The listing builds one solid part. Answer for the finished solid, in the listing's coordinates (mm). Face numbers are marked on the shaded views. Round coordinates to 2 decimals unless told otherwise and drop trailing zeros. Order: outer loops, then holes, each group sorted by start corner. A loop starts at its lowest first (then second) coordinate and runs counter-clockwise, first axis right, second up. Notation, with made-up numbers: (86, 72.25) - (104, 72.25) arc R26 ccw to (104, 101.25) - close; hole circle Ø4 at (51.25, 25). An arc over 180 degrees is marked (long way). Write item = value, one per line.
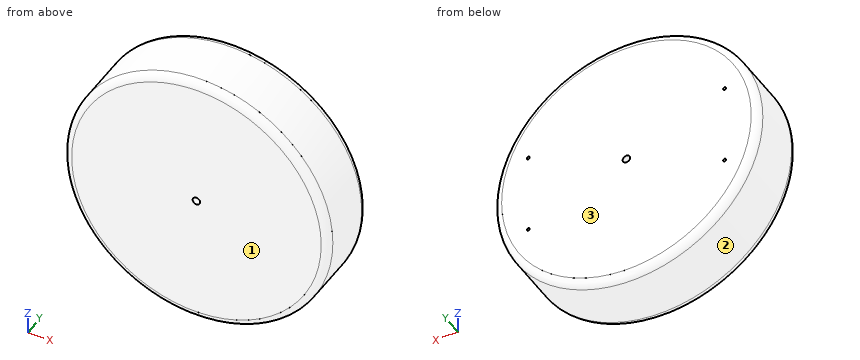
from build123d import *

# Parameters (mm, degrees)
SKETCH1_R           = 177
SKETCH1_R_2         = 5
BOSS_EXTRUDE1_DEPTH = 89
SKETCH2_R           = 1.975
CUT_EXTRUDE1_DEPTH  = 19
FILLET1_R           = 10


with BuildPart() as part:
    # Sketch1 → Boss-Extrude1 (new body)
    with BuildSketch(Plane(origin=(0, 0, 0), x_dir=(1, 0, 0), z_dir=(0, 1, 0))):
        Circle(SKETCH1_R)
        Circle(SKETCH1_R_2, mode=Mode.SUBTRACT)
    extrude(amount=BOSS_EXTRUDE1_DEPTH)

    # Sketch2 → Cut-Extrude1 (cut)
    with BuildSketch(Plane(origin=(0, 89, 0), x_dir=(1, 0, 0), z_dir=(0, 1, 0))):
        with Locations((-131.4, 53.9)):
            Circle(SKETCH2_R)
        with Locations((-131.4, -53.9)):
            Circle(SKETCH2_R)
        with Locations((131.4, -53.9)):
            Circle(SKETCH2_R)
        with Locations((131.4, 53.9)):
            Circle(SKETCH2_R)
    extrude(amount=-CUT_EXTRUDE1_DEPTH, mode=Mode.SUBTRACT)

    # Fillet1
    fillet1_edges = [part.edges().sort_by_distance(p)[0] for p in [
        (-177, 0, 0),
        (-177, 89, 0),
    ]]
    fillet(fillet1_edges, radius=FILLET1_R)


solid = part.part
Q1. Flat-ended cylindrical pins translate along their axes: P1, Ø3.5, axis at x = 131.4, z = -53.9, coming from the +Y side; P2, Ø5, axis at y = 43.5, z = -113, coming from the -X side; P3, Ø1.5, axis at x = -109, y = 72, coming from the -Z side. Find the tip coordinate at first contact, or state that the pin passes through.
Model answer:
P1 = 70
P2 = -138.27
P3 = -140.04
Q2. Section A-A on y = 18.5 is taken. Determine the outline of the cut face in (x, z).
Model answer:
outline = circle Ø354 at (0, 0); hole circle Ø10 at (0, 0)
Q3. Find the intervals of material crossed by line 1 (X direction, y = 50.5, z = 0); line 2 (X direction, y = 81.5, z = 53.9) (3 decimals); line 3 (Z direction, x = 131, y = 80), in increasing order. Write a range as from..to.
Model answer:
line_1 = -177..-5, 5..177
line_2 = -168.26..-133.375, -129.425..129.425, 133.375..168.26
line_3 = -118.95..-55.83, -51.97..51.97, 55.83..118.95
Q4. Determine the mould class of the marked faces 1, 2 and 3 for opening direction Y: released by +Y, released by -Y, zero draft, split by the parting line, or undercut.
Model answer:
face_1 = released by -Y
face_2 = zero draft
face_3 = released by +Y
